Could you check a few things on this drawing? It's one solid part, dimensions in mm from its lowest x, y, z. A direction names the side the tool comes from. Coordinates: 2 decimals unless noted, no trailing zeros. Order: outer loops, then holes, each group sorted by start corner. A loop starts at its lowest first (then second) coordinate and runs counter-clockwise, first axis right, second up. Notation, with made-up numbers: (-22.5, 52) -> (25.5, 52) arc R22 cw to (25.5, 88) -> close; hole circle Ø4 at (10, 71.25). An arc over 180 degrees is marked (long way). Use a Markdown table: item, result. Add a question column.
1. If I drill on line 1 along X through (y, z) = (60, 24.75), over which ranges is the centre line in solid material (lowest first)? Write a range as from..to.
2. We'd pull the mould along Z, two halves only. Please class the marked faces 1, 2 and 3: pulls with the +Z half, pulls with the -Z half, needs draft (parallel to the pull), parting line crosses it, or undercut.
3. Suppose I cut it at B-B, the plane z = 7.25. List the corners of the cut face in (x, y) for me.
4. Suppose I cut it at A-A, the plane x = 11.25. List the corners of the cut face in (y, z) for me.
5. Suppose I cut it at C-C, the plane y = 49.5. List the corners of the cut face in (x, z) for me.
6. For the marked faces 4 and 5, which set-ups out of +Z, -Z, +X, -X, +Y, -Y let a thin tool reach every point of the face, with its end or its side?
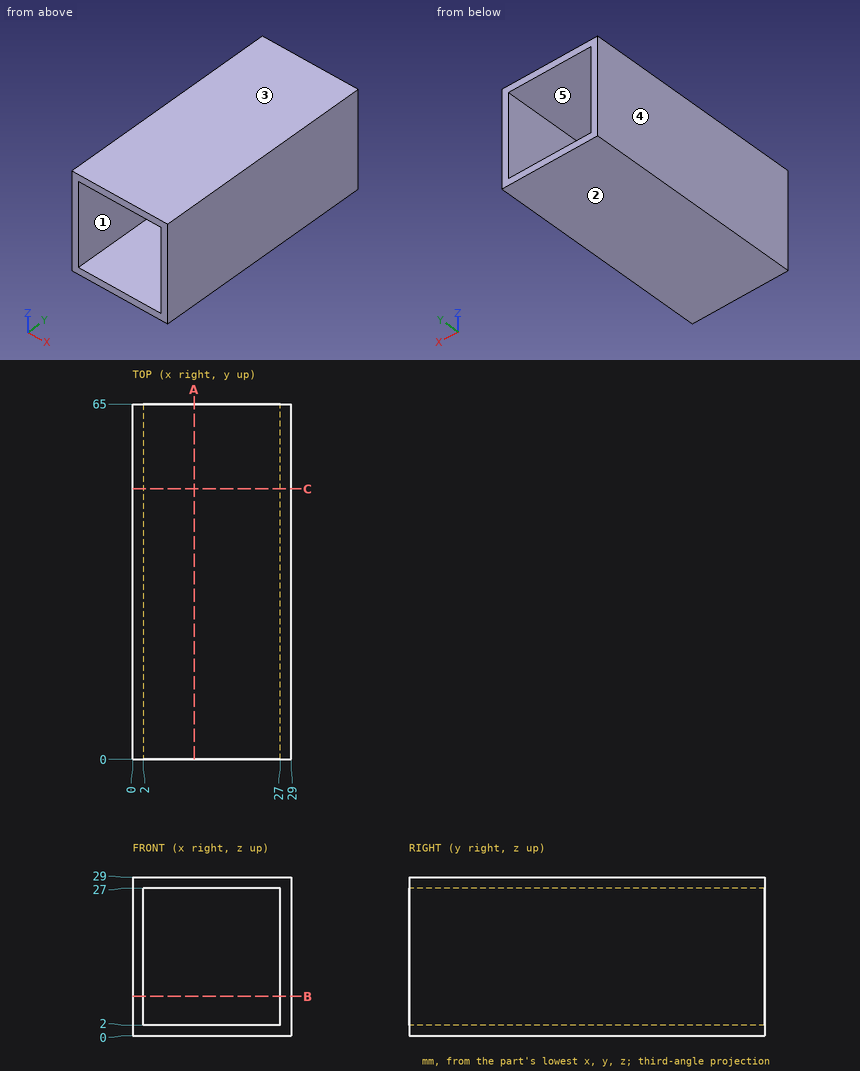
Worked out:
| question | item | result |
|---|---|---|
| 1 | line 1 | x = 0..2, 27..29 |
| 2 | face 1 | undercut |
| 2 | face 2 | pulls with the -Z half |
| 2 | face 3 | pulls with the +Z half |
| 3 | outline | (0, 0) -> (2, 0) -> (2, 65) -> (0, 65) -> close; (27, 0) -> (29, 0) -> (29, 65) -> (27, 65) -> close |
| 4 | outline | (0, 0) -> (65, 0) -> (65, 2) -> (0, 2) -> close; (0, 27) -> (65, 27) -> (65, 29) -> (0, 29) -> close |
| 5 | outline | (0, 0) -> (29, 0) -> (29, 29) -> (0, 29) -> close; hole (2, 2) -> (27, 2) -> (27, 27) -> (2, 27) -> close |
| 6 | face 4 | +Z, -Z, -X, +Y, -Y |
| 6 | face 5 | +Y, -Y |
